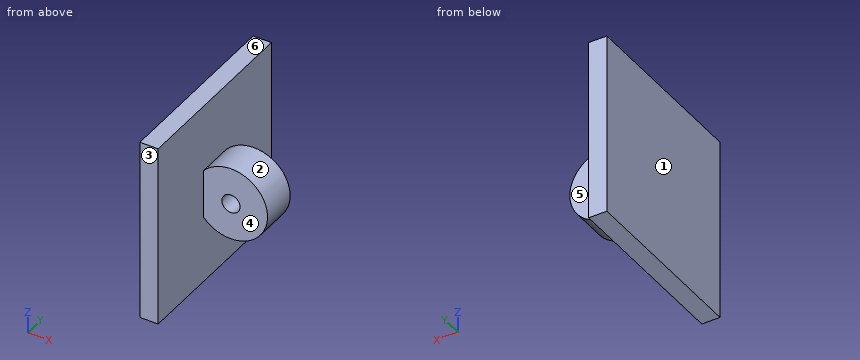
from build123d import *

# Parameters (mm, degrees)
F0_W     = 100
F0_H     = 100
F1_DEPTH = 10
F2_W     = 20
F2_H     = 70
F3_DEPTH = 70
F5_DEPTH = 60.001
F4_R     = 5
F6_DEPTH = 60.001


with BuildPart() as f1:
    # F0 (on Right) → F1 (new body)
    with BuildSketch(Plane.YZ):
        Rectangle(F0_W, F0_H)
    extrude(amount=F1_DEPTH)

    # F2 (on face) → F3 (join)
    with BuildSketch(Plane.YZ.offset(10)):
        Rectangle(F2_W, F2_H)
    extrude(amount=F3_DEPTH)

    # F4 (on face) → F5 (cut, through all)
    with BuildSketch(Plane(origin=(0, 10, 0), x_dir=(-1, 0, 0), z_dir=(0, 1, 0))):
        with BuildLine():
            ThreePointArc((-10, -13.228757), (-45, 0), (-10, 13.228757))
            Line((-10, 13.228757), (-10, 35))
            Line((-10, 35), (-80, 35))
            Line((-80, 35), (-80, -35))
            Line((-80, -35), (-10, -35))
            Line((-10, -35), (-10, -13.228757))
        make_face()
    extrude(amount=-F5_DEPTH, mode=Mode.SUBTRACT)

    # F4 (on face) → F6 (cut, through all)
    with BuildSketch(Plane(origin=(0, 10, 0), x_dir=(-1, 0, 0), z_dir=(0, 1, 0))):
        with Locations((-25, 0)):
            Circle(F4_R)
    extrude(amount=-F6_DEPTH, mode=Mode.SUBTRACT)


solid = f1.part
Can you work these out from the model? Positions are in its coordinate system, mm. Face numbers are marked on the shaded views. A direction names the side the tool comes from. Give positions to 0.01 mm unless a question says otherwise; leave off trailing zeros. Order: outer loops, then holes, each group sorted by start corner. A loop starts at its lowest first (then second) coordinate and runs counter-clockwise, first axis right, second up. Notation, with made-up numbers: M 52.25,-16.5 L 89.25,-16.5 A19 cw 89.25,15.5 Z; hole C 46,29 d6. An arc over 180 degrees is marked long. Use one line per item in the form item = value. Start each with the question number.
Item 1: For the marked faces 4, 5 and 6, which set-ups out of +Z, -Z, +X, -X, +Y, -Y let a thin tool reach every point of the face, with its end or its side?
Item 2: If we section it at C-C (y = -0.5): Write out the boundary of the cut face in (x, z).
Item 3: Will these pins go through, and if not, where does the flat tip stop? pin 1 Ø8 at (x, z) = (27.5, -19.5) entering from +Y; pin 2 Ø1 at (y, z) = (-17, -1) entering from -X; pin 3 Ø4 at (y, z) = (2.5, -29.5) entering from +X.
Item 4: We'd pull the mould along X, two halves only. Please class the marked faces 1, 2 and 3: +X half, -X half, draft (parallel to the pull), parting line (faces both ways), or undercut.
Item 5: If I drill on line 1 along Z through (x, y) = (25, -2); line 2 along Y through (x, z) = (28.5, -10); line 3 along X through (y, z) = (37, 0), over which ranges is the centre line in solid material (lowest first)?
Item 6: If we section it at B-B (x = 25): Write out the boundary of the cut face in (y, z), then the cut area to 3 significant figures.
Item 7: If we section it at A-A (z = 0): Write out the boundary of the cut face in (x, y), then the cut area to 3 significant figures.
Item 8: If we section it at D-D (z = -36): Write out the boundary of the cut face in (x, y), then the cut area to 3 significant figures.
Outcome:
q1.face_4 = +Z, -Z, +X, -Y
q1.face_5 = +Z, -Z, +X, +Y
q1.face_6 = +Z, +X, -X, +Y, -Y
q2.outline = M 0,-50 L 10,-50 L 10,-13.23 A20 ccw long 10,13.23 L 10,50 L 0,50 Z; hole C 25,0 d10
q3.pin_1 = 10
q3.pin_2 = 0
q3.pin_3 = 10
q4.face_1 = -X half
q4.face_2 = undercut
q4.face_3 = draft
q5.line_1 = -20 to -5, 5 to 20
q5.line_2 = -10 to 10
q5.line_3 = 0 to 10
q6.outline = M -10,-20 L 10,-20 L 10,-5 L -10,-5 Z; M -10,5 L 10,5 L 10,20 L -10,20 Z
q6.area = 600 mm2
q7.outline = M 0,-50 L 10,-50 L 10,-10 L 20,-10 L 20,10 L 10,10 L 10,50 L 0,50 Z; M 30,-10 L 45,-10 L 45,10 L 30,10 Z
q7.area = 1,500 mm2
q8.outline = M 0,-50 L 10,-50 L 10,50 L 0,50 Z
q8.area = 1,000 mm2
